Check sheet for the modelled part. Datum: model origin and axes. Units: mm. A direction names the side the tool comes from. Round coordinates to 2 decimals unless told otherwise and drop trailing zeros. Write each loop counter-clockwise with the first axis right and the second up, starting at its lowest first coordinate (ties: lowest second). Pieces come first, ordered by that corner, then holes. Notation, with made-up numbers: (-18, 54) -> (11, 54) arc R20 ccw to (11, 87) -> close; hole circle Ø7 at (12, 72.5). An arc over 180 degrees is marked (long way). Answer as a JSON object with one key per item and string values. Group by question number.
```python
from build123d import *

# Parameters (mm, degrees)
SKETCH2_W           = 3.6
SKETCH2_H           = 2
BOSS_EXTRUDE1_DEPTH = 7


with BuildPart() as part:
    # Sketch1 → Revolve1 (revolve)
    with BuildSketch(Plane(origin=(0, 0, 0), x_dir=(0, 0, -1), z_dir=(1, 0, 0)), mode=Mode.PRIVATE) as revolve1_sk:
        Polygon((6.5, 2.75), (12, 1.5), (12, 0.9), (-12, 0.9), (-12, 1.5), (-6.5, 2.75), (-6.5, 2.15), (-3.9, 2.15), (-2, 2.55), (-2, 4.55), (-1, 4.55), (-1, 3.05), (1, 3.05), (1, 4.55), (2, 4.55), (2, 2.55), (3.9, 2.15), (6.5, 2.15), align=None)
    revolve(revolve1_sk.sketch.rotate(Axis((0, 0, 12), (0, 0, -1)), 180), axis=Axis((0, 0, 12), (0, 0, -1)))

    # Sketch2 → Boss-Extrude1 (add)
    with BuildSketch(Plane(origin=(0, 0, 0), x_dir=(1, 0, 0), z_dir=(0, 1, 0))):
        Polygon((-4.55, 2), (-4.55, 1), (-2.8, 1), (-2.8, -1), (-4.55, -1), (-4.55, -2), (4.55, -2), (4.55, -1), (2.8, -1), (2.8, 1), (4.55, 1), (4.55, 2), align=None)
        Rectangle(SKETCH2_W, SKETCH2_H, mode=Mode.SUBTRACT)
    extrude(amount=BOSS_EXTRUDE1_DEPTH)


solid = part.part
```
(1) Scan lines: line 1 along Z through (x, y) = (1.75, 4); line 2 along X through (y, z) = (0, 5.5); line 3 along Z through (x, y) = (-2, 4.75). Record each from-to range of solid material in increasing order.
(2) Section check A-A on y = 5.75. Record the cut outline in (x, z), then the cut area to 3 significant figures.
(3) Section check B-B on z = 8.75. Record the cut outline in (x, y), then the cut area to 3 significant figures.
(4) Access from +Z, -Z, +X, -X, +Y, -Y to the whole of each face (thin tool, end or side, straight path). Record for faces 4 (the flat face through (-2.8, 4, 0)), 5 (the flat face through (0, 5, 1)), 6 (the flat face through (-3.1, 1.1, -1)).
(5) Go/stop test with flat-tipped pins: pin 1 Ø4 at (x, z) = (0.5, 6.5) entering from +Y; pin 2 Ø2 at (x, y) = (2, 4) entering from +Z; pin 3 Ø1.6 at (y, z) = (5, 0) entering from +X. Record where each tip stops, or that it passes through.
(6) Section check C-C on z = -3. Record the cut outline in (x, y).
(7) Release check for a two-part mould opening along X. For faces 1 (the cylindrical face through (0.1, -4.55, 1.49)), 2 (the flat face through (0, 0, -1.5)), 3 (the flat face through (-4.55, 3.5, 1.5)) record: pulls with the +X half, pulls with the -X half, needs draft (parallel to the pull), parting line crosses it, or undercut.
Data:
{
 "1": {"line 1": "z = -2 to -1, 1 to 2", "line 2": "x = -2.15 to -0.9, 0.9 to 2.15", "line 3": "z = -2 to 2"},
 "2": {"outline": "(-4.55, -2) -> (4.55, -2) -> (4.55, -1) -> (2.8, -1) -> (2.8, 1) -> (4.55, 1) -> (4.55, 2) -> (-4.55, 2) -> (-4.55, 1) -> (-2.8, 1) -> (-2.8, -1) -> (-4.55, -1) -> close; hole (-1.8, -1) -> (1.8, -1) -> (1.8, 1) -> (-1.8, 1) -> close", "area": "22.2 mm²"},
 "3": {"outline": "circle Ø4.48 at (0, 0); hole circle Ø1.8 at (0, 0)", "area": "13.2 mm²"},
 "4": {"face 4": "-X, +Y", "face 5": "+Y", "face 6": "none"},
 "5": {"pin 1": "stops at y = 2.75", "pin 2": "stops at z = 2", "pin 3": "stops at x = 2.8"},
 "6": {"outline": "circle Ø4.68 at (0, 0); hole circle Ø1.8 at (0, 0)"},
 "7": {"face 1": "parting line crosses it", "face 2": "undercut", "face 3": "pulls with the -X half"}
}
